Read the model definition and answer for the solid it produces. Units are mm, in the model's axes. A direction names the side the tool comes from. Coordinates: 2 decimals unless noted, no trailing zeros. Loops run counter-clockwise (first coordinate to the right, second up) from the corner with the lowest first, then second, coordinate; pieces in that order, holes last. Notation, with made-up numbers: M -15,5 L 2,5 A18 ccw 2,28 Z; hole C 3.25,-35.75 d5. An arc over 180 degrees is marked long. One line per item, written item: value. Start each with the question number.
1. Determine the mould class of faces 1 (the face through (-4, 14, 44)), 2 (the face through (-32, 24, -20)), 3 (the face through (0, 0, -44)) for opening direction Y: +Y half, -Y half, draft (parallel to the pull), parting line (faces both ways), or undercut.
2. Consider probe 1 along X at (y, z) = (3.25, 1.5); probe 2 along Z at (x, y) = (-50, 13.5); probe 3 along Z at (x, y) = (34.5, 23.25). Determine where each line is inside the solid, lowest interval first.
3. The part is cut by section D-D (x = -37). Write down the section's boundary in (y, z), then the cut area to 4 significant figures.
4. A flat-ended cylindrical pin translates along its axis: pin 1 (25 mm diameter, centred on x = 25.5, z = -20, fed in from -Y). Find the tip coordinate at first contact, or state that the pin passes through.
5. The part is cut by section A-A (x = 46). Write down the section's boundary in (y, z), then the cut area to 4 significant figures.
6. The part is cut by section C-C (y = 20.25). Write down the section's boundary in (x, z).
7. For faces 4 (the face through (31, 24, -31)), 5 (the face through (-0.8, 9.5, 45)), 6 (the face through (-1, 12, -42)), determine the directions among +Z, -Z, +X, -X, +Y, -Y from which every point of the face is accessible in a straight line to the end or side of a thin tool.
8. The part is cut by section B-B (z = -26). Write down the section's boundary in (x, y), then the cut area to 4 significant figures.
```python
from build123d import *

# Parameters (mm, degrees)
SKETCH1_W           = 120
SKETCH1_H           = 90
BOSS_EXTRUDE1_DEPTH = 25
SKETCH2_W           = 114
SKETCH2_H           = 84
CUT_EXTRUDE1_DEPTH  = 22
SKETCH3_W           = 117
SKETCH3_H           = 87
CUT_EXTRUDE2_DEPTH  = 1.5
CUT_EXTRUDE3_DEPTH  = 11.5
SKETCH5_W           = 8
SKETCH5_H           = 8
CUT_EXTRUDE4_DEPTH  = 11.5
SKETCH6_R           = 0.4
CUT_EXTRUDE6_DEPTH  = 21.5


with BuildPart() as part:
    # Sketch1 → Boss-Extrude1 (new body)
    with BuildSketch(Plane(origin=(0, 0, 0), x_dir=(1, 0, 0), z_dir=(0, 1, 0))):
        Rectangle(SKETCH1_W, SKETCH1_H)
    extrude(amount=BOSS_EXTRUDE1_DEPTH)

    # Sketch2 → Cut-Extrude1 (cut)
    with BuildSketch(Plane.XZ):
        Rectangle(SKETCH2_W, SKETCH2_H)
    extrude(amount=-CUT_EXTRUDE1_DEPTH, mode=Mode.SUBTRACT)

    # Sketch3 → Cut-Extrude2 (cut)
    with BuildSketch(Plane.XZ):
        Rectangle(SKETCH3_W, SKETCH3_H)
    extrude(amount=-CUT_EXTRUDE2_DEPTH, mode=Mode.SUBTRACT)

    # Sketch4 → Cut-Extrude3 (cut)
    with BuildSketch(Plane(origin=(0, 25, 0), x_dir=(1, 0, 0), z_dir=(0, 1, 0))):
        Polygon((28, 31), (35, 31), (35, 36), (43, 36), (43, 31), (50, 31), (50, 20), (28, 20), align=None)
        Polygon((-50, 31), (-50, 20), (-43, 20), (-43, 15), (-35, 15), (-35, 20), (-28, 20), (-28, 31), align=None)
    extrude(amount=-CUT_EXTRUDE3_DEPTH, mode=Mode.SUBTRACT)

    # Sketch5 → Cut-Extrude4 (cut)
    with BuildSketch(Plane.XY.offset(45)):
        with Locations((0, 14)):
            Rectangle(SKETCH5_W, SKETCH5_H)
    extrude(amount=-CUT_EXTRUDE4_DEPTH, mode=Mode.SUBTRACT)

    # Sketch6 → Cut-Extrude6 (cut)
    with BuildSketch(Plane(origin=(0, 25, 0), x_dir=(1, 0, 0), z_dir=(0, 1, 0))):
        with Locations((-4.59237925, -11.959320964)):
            Circle(SKETCH6_R)
        with Locations((-1.19237925, -11.959320964)):
            Circle(SKETCH6_R)
    extrude(amount=-CUT_EXTRUDE6_DEPTH, mode=Mode.SUBTRACT)


solid = part.part
```
Answer block:
1. face 1: undercut
1. face 2: draft
1. face 3: -Y half
2. probe 1: x = -60 to -57, 57 to 60
2. probe 2: z = -45 to -42, 42 to 45
2. probe 3: z = -45 to -31, -20 to 45
3. outline: M 0,-45 L 25,-45 L 25,-31 L 22,-31 L 22,-42 L 1.5,-42 L 1.5,-43.5 L 0,-43.5 Z; M 0,43.5 L 1.5,43.5 L 1.5,42 L 22,42 L 22,-15 L 25,-15 L 25,45 L 0,45 Z
3. area: 349.5 mm2
4. pin 1: stops at y = 22
5. outline: M 0,-45 L 25,-45 L 25,-31 L 22,-31 L 22,-42 L 1.5,-42 L 1.5,-43.5 L 0,-43.5 Z; M 0,43.5 L 1.5,43.5 L 1.5,42 L 22,42 L 22,-20 L 25,-20 L 25,45 L 0,45 Z
5. area: 364.5 mm2
6. outline: M -60,-45 L 60,-45 L 60,45 L -60,45 Z; hole M -57,-42 L 57,-42 L 57,42 L -57,42 Z
7. face 4: +Y, -Y
7. face 5: +Z, +X, -X, +Y, -Y
7. face 6: -Y
8. outline: M -60,0 L -58.5,0 L -58.5,1.5 L -57,1.5 L -57,22 L -50,22 L -50,25 L -60,25 Z; M -28,22 L 28,22 L 28,25 L -28,25 Z; M 50,22 L 57,22 L 57,1.5 L 58.5,1.5 L 58.5,0 L 60,0 L 60,25 L 50,25 Z
8. area: 355.5 mm2
